Study the drawing (mm; zero at the part's minimum x, y, z) and answer. A direction names the side the tool comes from. Coordinates: 2 decimals unless noted, no trailing zeros. Write each loop counter-clockwise with the first axis right and the second up, starting at its lowest first coordinate (ties: lowest second). Pieces come first, ordered by that corner, then holes. Notation, with made-up numbers: (52.5, -19) - (68.5, -19) arc R24 ccw to (68.5, -7) - close; hole circle Ø9 at (0.25, -27.5). An arc over 180 degrees is marked (long way). One line per item, written item: value.
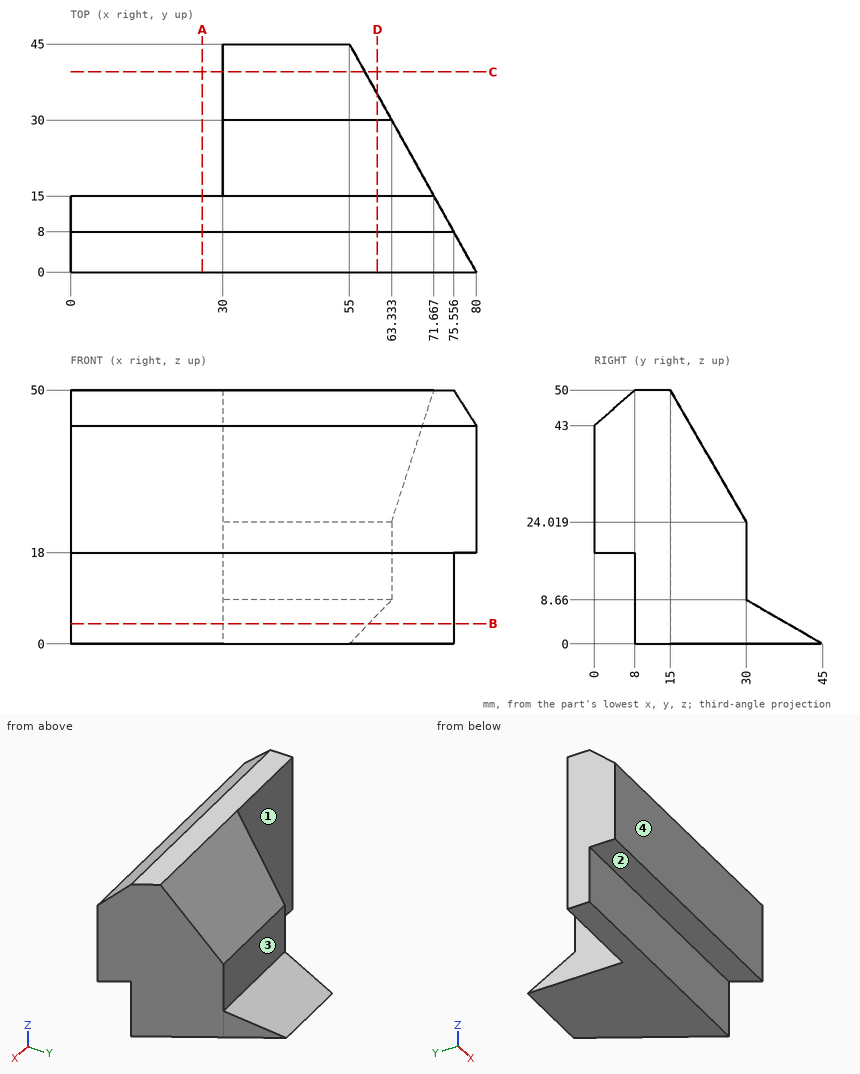
Item 1: Section C-C, the plane y = 39.5 is taken. Determine the outline of the cut face in (x, z) (1 decimal).
Evaluation:
outline: (30, 0) - (58.1, 0) - (58.1, 3.2) - (30, 3.2) - close
Item 2: Consider probe 1 along Y at (x, z) = (17, 41); probe 2 along Y at (x, z) = (25, 3); probe 3 along X at (y, z) = (10, 19) (1 decimal). Determine where each line is inside the solid, lowest interval first.
Evaluation:
probe 1: y = 0 to 15
probe 2: y = 8 to 15
probe 3: x = 0 to 74.4
Item 3: Section D-D, the plane x = 60.5 is taken. Determine the outline of the cut face in (y, z) (1 decimal), then the cut area to 3 significant figures.
Evaluation:
outline: (0, 18) - (8, 18) - (8, 0) - (35.1, 0) - (35.1, 5.7) - (30, 8.7) - (30, 24) - (15, 50) - (8, 50) - (0, 43) - close
area: 1,170 mm2
Item 4: Section A-A, the plane x = 26 is taken. Determine the outline of the cut face in (y, z).
Evaluation:
outline: (0, 18) - (8, 18) - (8, 0) - (15, 0) - (15, 50) - (8, 50) - (0, 43) - close
Item 5: Which of the six approach directions +Z, -Z, +X, -X, +Y, -Y give full straight-line access (tool end or side, diameter ignored) to the marked faces 1, 2, 3 and 4?
Evaluation:
face 1: +Z, -Z, -X, +Y
face 2: -Z, +X, -X, -Y
face 3: +Z, +X, -X, +Y
face 4: +Z, -Z, +X, -X, -Y
Item 6: Section B-B, the plane z = 4 is taken. Determine the outline of the cut face in (x, y) (1 decimal), then the cut area to 3 significant figures.
Evaluation:
outline: (0, 8) - (75.6, 8) - (58.8, 38.1) - (30, 38.1) - (30, 15) - (0, 15) - close
area: 1,330 mm2
Item 7: Given pin 1 (9 mm diameter, centred on y = 24.5, z = 14, fed in from -X); pin 2 (20 mm diameter, centred on x = 20, z = 7, fed in from -Y); pin 3 (2.5 mm diameter, centred on x = 23.5, y = 5, fed in from -Z), each flat-ended and moving along its own axis, determine where each tip first touches the part or whether it passes through.
Evaluation:
pin 1: stops at x = 30
pin 2: stops at y = 8
pin 3: stops at z = 18
